Could you check a few things on this drawing? It's one solid part, dimensions in mm from its lowest x, y, z. A direction names the side the tool comes from. Give positions to 0.01 mm unless a question says otherwise; leave off trailing zeros. Loops run counter-clockwise (first coordinate to the right, second up) from the corner with the lowest first, then second, coordinate; pieces in that order, holes last. Notation, with made-up numbers: (-37, -31.75) - (1, -31.75) arc R14 cw to (1, -4.75) - close; hole circle Ø11 at (24.5, 20). An arc over 180 degrees is marked (long way). Answer as a JSON object with one key per item and string values.
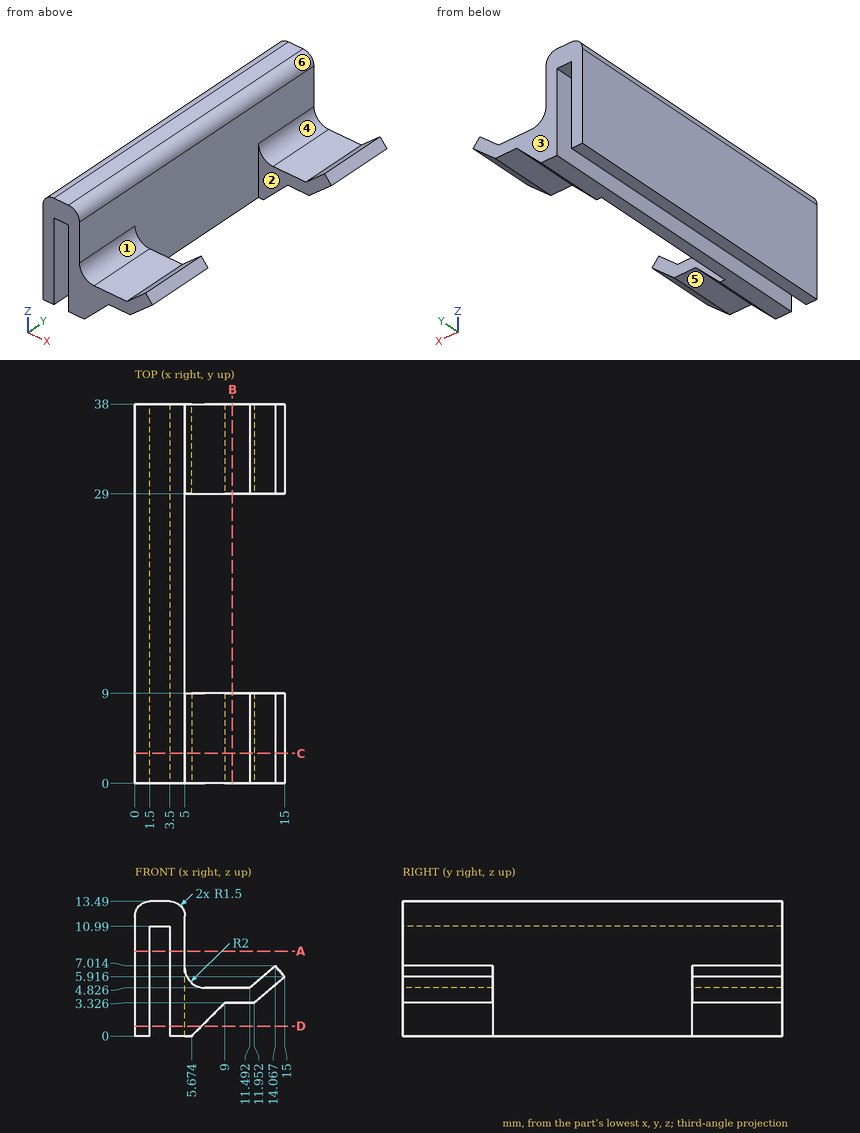
1) Which directions (+Z, -Z, +X, -X, +Y, -Y) give clear straight access to the entire face, cutting with the end or side of a thin tool? Please do the marked faces 4, 5 and 6.
Check sheet entries:
{"face 4": "+Z, +Y, -Y", "face 5": "-Z, +X, +Y, -Y", "face 6": "+Z, +X, +Y, -Y"}
2) I'm going to push flat-ended pins straight in: P1, Ø8, axis at x = 12.5, y = 14.5, coming from the +Z side; P2, Ø5, axis at x = 8.5, y = 34.5, coming from the +Z side; P3, Ø1.5, axis at x = 11, y = 6, coming from the -Z side; P4, Ø6, axis at y = 19.5, z = 9, coming from the +X side. Where does each tip first touch, or does it pass through?
Check sheet entries:
{"P1": "through", "P2": "z = 5.09", "P3": "z = 3.33", "P4": "x = 5"}
3) Imagine slicing it at D-D on z = 1. Write out the boundary of the cut face in (x, y) (1 decimal).
Check sheet entries:
{"outline": "(0, 0) - (1.5, 0) - (1.5, 38) - (0, 38) - close; (3.5, 0) - (6.7, 0) - (6.7, 9) - (5, 9) - (5, 29) - (6.7, 29) - (6.7, 38) - (3.5, 38) - close"}
4) If we mould it in two halves opening along Y, with no side actions, what happens to the marked faces 1, 2 and 3? For each: released by +Y, released by -Y, zero draft, split by the parting line, or undercut.
Check sheet entries:
{"face 1": "zero draft", "face 2": "undercut", "face 3": "released by +Y"}
5) I need wall thicknesses on L1, parallel to X at y = 12.5, z = 9.75; L2, parallel to Y at x = 10.5, z = 4.75; L3, parallel to X at y = 5.5, z = 6.75 (1 decimal). Which ranges of each line are inside material? Lowest first, please.
Check sheet entries:
{"L1": "0 to 1.5, 3.5 to 5", "L2": "0 to 9, 29 to 38", "L3": "0 to 1.5, 3.5 to 5, 13.8 to 14.3"}
6) Imagine slicing it at C-C on y = 3. Write out the boundary of the cut face in (x, z) (1 decimal).
Check sheet entries:
{"outline": "(0, 0) - (1.5, 0) - (1.5, 11) - (3.5, 11) - (3.5, 0) - (5.7, 0) - (9, 3.3) - (12, 3.3) - (15, 5.9) - (14.1, 7) - (11.5, 4.8) - (7, 4.8) arc R2 cw to (5, 6.8) - (5, 12) arc R1.5 ccw to (3.5, 13.5) - (1.5, 13.5) arc R1.5 ccw to (0, 12) - close"}
7) Imagine slicing it at B-B on x = 9.75. Write out the boundary of the cut face in (y, z) (1 decimal), and give its area (3 significant figures).
Check sheet entries:
{"outline": "(0, 3.3) - (9, 3.3) - (9, 4.8) - (0, 4.8) - close; (29, 3.3) - (38, 3.3) - (38, 4.8) - (29, 4.8) - close", "area": "27.0 mm2"}
8) Imagine slicing it at A-A on z = 8.5. Write out the boundary of the cut face in (x, y).
Check sheet entries:
{"outline": "(0, 0) - (1.5, 0) - (1.5, 38) - (0, 38) - close; (3.5, 0) - (5, 0) - (5, 38) - (3.5, 38) - close"}
